Here's how the part is built. I have some questions about the finished solid (model axes, mm). A direction names the side the tool comes from. Coordinates: 2 decimals unless noted, no trailing zeros. Write each loop counter-clockwise with the first axis right and the second up, starting at its lowest first coordinate (ties: lowest second). Pieces come first, ordered by that corner, then holes. Notation, with made-up numbers: M 25.5,-34.75 L 76.5,-34.75 A15 ccw 76.5,-8.75 Z; hole C -0.75,-27 d11. An arc over 180 degrees is marked long. Write each question's results on one line, items separated by ' | '. Start each with the question number.
from build123d import *

# Parameters (mm, degrees)
SKETCH1_W           = 70
SKETCH1_H           = 200
BOSS_EXTRUDE4_DEPTH = 15
SKETCH9_R           = 6
CUT_EXTRUDE1_DEPTH  = 71
BOSS_EXTRUDE5_DEPTH = 33


with BuildPart() as part:
    # Sketch1 → Boss-Extrude4 (new body)
    with BuildSketch(Plane.XY):
        Rectangle(SKETCH1_W, SKETCH1_H)
    extrude(amount=BOSS_EXTRUDE4_DEPTH)

    # Sketch9 → Cut-Extrude1 (cut, through all)
    with BuildSketch(Plane(origin=(35, 0, 0), x_dir=(0, 0, -1), z_dir=(1, 0, 0))):
        with Locations((-7.5, -85)):
            Circle(SKETCH9_R)
    extrude(amount=-CUT_EXTRUDE1_DEPTH, mode=Mode.SUBTRACT)

    # Sketch10 → Boss-Extrude5 (add)
    with BuildSketch(Plane(origin=(0, 100, 0), x_dir=(1, 0, 0), z_dir=(0, 1, 0))):
        with BuildLine():
            Line((31.622776602, -15), (-31.622776602, -15))
            ThreePointArc((-31.622776602, -15), (0, -35), (31.622776602, -15))
        make_face()
    extrude(amount=-BOSS_EXTRUDE5_DEPTH)


solid = part.part
1) Please list where these lines run through material, in increasing order: line 1 (Y direction, x = 3, z = 7.5); line 2 (Z direction, x = -32, y = -26.5); line 3 (Y direction, x = 5, z = 24). Write a range as [from, to].
2) We'd pull the mould along Z, two halves only. Please class faces 3 (the flat face through (0, 1, 0)), 4 (the flat face through (0, 100, 13)), 5 (the cylindrical face through (0.49, -79.05, 8.28)), 6 (the cylindrical face through (-0.553, 83.731, 34.996)): pulls with the +Z half, pulls with the -Z half, needs draft (parallel to the pull), parting line crosses it, or undercut.
3) I want a section at A-A, the plane z = 7.5. Write out the boundary of the cut face in (x, y), then the cut area to 3 significant figures.
4) I want a section at D-D, the plane x = 18. Write out the boundary of the cut face in (y, z).
5) For faces 1 (the flat face through (0, -100, 7)), 2 (the flat face through (0, 67, 23)), which set-ups out of +Z, -Z, +X, -X, +Y, -Y let a thin tool reach every point of the face, with its end or its side?
6) I want a section at B-B, the plane y = -85. Write out the boundary of the cut face in (x, z), then the cut area to 3 significant figures.
7) I want a section at C-C, the plane x = 3.5. Write out the boundary of the cut face in (y, z), then the cut area to 3 significant figures.
8) For pin 1 Ø10 at (x, y) = (-8.5, -59) entering from +Z; pin 2 Ø10 at (x, z) = (27, 22) entering from -Y, each with a flat end and sliding along its axis, tell me the tip position at first contact or that it passes through.
Output:
1) line 1: y = [-100, -91], [-79, 100] | line 2: z = [0, 15] | line 3: y = [67, 100]
2) face 3: pulls with the -Z half | face 4: needs draft | face 5: undercut | face 6: pulls with the +Z half
3) outline: M -35,-100 L 35,-100 L 35,-91 L -35,-91 Z; M -35,-79 L 35,-79 L 35,100 L -35,100 Z | area: 13,200 mm2
4) outline: M -100,0 L 100,0 L 100,30.02 L 67,30.02 L 67,15 L -100,15 Z; hole C -85,7.5 d12
5) face 1: +Z, -Z, +X, -X, -Y | face 2: +Z, +X, -X, -Y
6) outline: M -35,0 L 35,0 L 35,1.5 L -35,1.5 Z; M -35,13.5 L 35,13.5 L 35,15 L -35,15 Z | area: 210 mm2
7) outline: M -100,0 L 100,0 L 100,34.82 L 67,34.82 L 67,15 L -100,15 Z; hole C -85,7.5 d12 | area: 3,540 mm2
8) pin 1: stops at z = 15 | pin 2: stops at y = 67
